Verification items for the finished model (mm, model axes). Face numbers are marked on the shaded views. A direction names the side the tool comes from. Give positions to 0.01 mm unless a question says otherwise; leave off trailing zeros. Write each loop counter-clockwise with the first axis right and the second up, starting at its lowest first coordinate (ties: lowest second). Pieces come first, ordered by that corner, then holes. Notation, with made-up numbers: M 88,78 L 135,78 A33 cw 135,106 Z; hole C 27.25,-36 d3. An arc over 180 degrees is marked long. Answer as a JSON object with one key per item and string values.
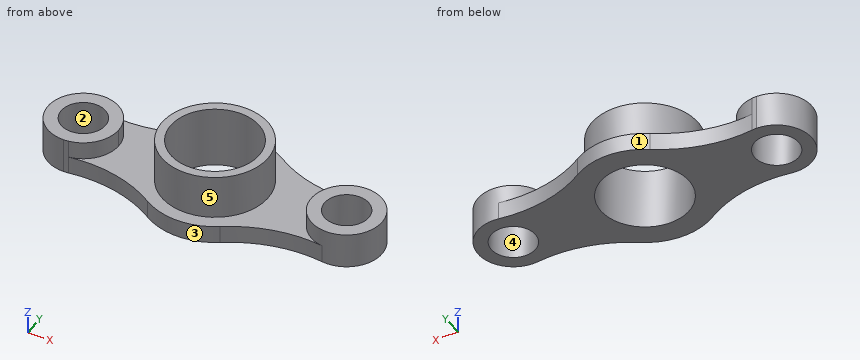
```python
from build123d import *

# Parameters (mm, degrees)
SKETCH1_R           = 60
BOSS_EXTRUDE1_DEPTH = 20
SKETCH1_3_R         = 60
SKETCH1_3_R_2       = 50
BOSS_EXTRUDE2_DEPTH = 70
SKETCH1_5_R         = 25
SKETCH1_5_R_2       = 40
BOSS_EXTRUDE3_DEPTH = 40


with BuildPart() as part:
    # Sketch1 → Boss-Extrude1 (new body)
    with BuildSketch(Plane.XY):
        with BuildLine():
            ThreePointArc((-144.403508772, -39.606556098), (-90.666225841, -41.750102304), (-41.138888889, -62.710380488))
            ThreePointArc((-41.138888889, -62.710380488), (0, -75), (41.138888889, -62.710380488))
            ThreePointArc((41.138888889, -62.710380488), (90.666225841, -41.750102304), (144.403508772, -39.606556098))
            ThreePointArc((144.403508772, -39.606556098), (110, 0), (144.403508772, 39.606556098))
            ThreePointArc((144.403508772, 39.606556098), (90.666225841, 41.750102304), (41.138888889, 62.710380488))
            ThreePointArc((41.138888889, 62.710380488), (0, 75), (-41.138888889, 62.710380488))
            ThreePointArc((-41.138888889, 62.710380488), (-90.666225841, 41.750102304), (-144.403508772, 39.606556098))
            ThreePointArc((-144.403508772, 39.606556098), (-119.801824152, 26.23109177), (-110, 0))
            ThreePointArc((-110, 0), (-119.801824152, -26.23109177), (-144.403508772, -39.606556098))
        make_face()
        Circle(SKETCH1_R, mode=Mode.SUBTRACT)
    extrude(amount=BOSS_EXTRUDE1_DEPTH)

    # Sketch1_3 → Boss-Extrude2 (add)
    with BuildSketch(Plane.XY):
        Circle(SKETCH1_3_R)
        Circle(SKETCH1_3_R_2, mode=Mode.SUBTRACT)
    extrude(amount=BOSS_EXTRUDE2_DEPTH)

    # Sketch1_5 → Boss-Extrude3 (add)
    # profile 1 of 2: a face of its own
    with BuildSketch(Plane.XY):
        with BuildLine():
            ThreePointArc((-150, -40), (-147.194847947, -39.90151779), (-144.403508772, -39.606556098))
            ThreePointArc((-144.403508772, -39.606556098), (-119.801824152, -26.23109177), (-110, 0))
            ThreePointArc((-110, 0), (-119.801824152, 26.23109177), (-144.403508772, 39.606556098))
            ThreePointArc((-144.403508772, 39.606556098), (-147.194847947, 39.90151779), (-150, 40))
            ThreePointArc((-150, 40), (-190, 0), (-150, -40))
        make_face()
        with Locations((-150, 0)):
            Circle(SKETCH1_5_R, mode=Mode.SUBTRACT)
    # profile 2 of 2: a face of its own
    with BuildSketch(Plane.XY):
        with Locations(Location((150, 0, 0), (0, 0, 98.042770343))):
            Circle(SKETCH1_5_R_2)
        with Locations((150, 0)):
            Circle(SKETCH1_5_R, mode=Mode.SUBTRACT)
    extrude(amount=BOSS_EXTRUDE3_DEPTH)


solid = part.part
```
1) Release check for a two-part mould opening along Y. For the marked faces 1, 2 and 3 record: pulls with the +Y half, pulls with the -Y half, needs draft (parallel to the pull), parting line crosses it, or undercut.
Completed:
{"face 1": "pulls with the +Y half", "face 2": "undercut", "face 3": "pulls with the -Y half"}
2) Thickness scan on L1, parallel to Y at x = -150, z = 29; L2, parallel to X at y = -29.5, z = 33; L3, parallel to Z at x = 60.5, y = 28. Record the ranges inside material, lowest first.
Completed:
{"L1": "y = -40 to -25, 25 to 40", "L2": "x = -177.01 to -122.99, -52.25 to -40.37, 40.37 to 52.25, 122.99 to 177.01", "L3": "z = 0 to 20"}
3) Section check A-A on x = 150. Record the boundary of the cut face in (y, z).
Completed:
{"outline": "M -40,0 L -25,0 L -25,40 L -40,40 Z; M 25,0 L 40,0 L 40,40 L 25,40 Z"}
4) Section check C-C on y = 45. Record the boundary of the cut face in (x, z), and give its area (3 significant figures).
Completed:
{"outline": "M -78.54,0 L -21.79,0 L -21.79,70 L -39.69,70 L -39.69,20 L -78.54,20 Z; M 21.79,0 L 78.54,0 L 78.54,20 L 39.69,20 L 39.69,70 L 21.79,70 Z", "area": "4,060 mm2"}
5) Go/stop test with flat-tipped pins: pin 1 (5 mm diameter, centred on y = 22.5, z = 40.5, fed in from -X); pin 2 (5 mm diameter, centred on y = 24.5, z = 28.5, fed in from -X); pin 3 (10 mm diameter, centred on y = -8, z = 23.5, fed in from -X). Record where each tip stops, or that it passes through.
Completed:
{"pin 1": "stops at x = -184.61", "pin 2": "stops at x = -183.41", "pin 3": "stops at x = -189.89"}
6) Section check B-B on z = 6.5. Record the boundary of the cut face in (x, y), and give its area (3 significant figures).
Completed:
{"outline": "M -144.4,-39.61 A150 cw -41.14,-62.71 A75 ccw 41.14,-62.71 A150 cw 144.4,-39.61 A40 ccw long 144.4,39.61 A150 cw 41.14,62.71 A75 ccw -41.14,62.71 A150 cw -144.4,39.61 A40 ccw long Z; hole C -150,0 d50; hole C 0,0 d100; hole C 150,0 d50", "area": "24,200 mm2"}
7) Section check D-D on z = 65. Record the boundary of the cut face in (x, y), and give its area (3 significant figures).
Completed:
{"outline": "C 0,0 d120; hole C 0,0 d100", "area": "3,460 mm2"}
8) Access from +Z, -Z, +X, -X, +Y, -Y to the whole of each face (thin tool, end or side, straight path). Record for the marked faces 4 and 5.
Completed:
{"face 4": "+Z, -Z", "face 5": "+Z"}
